```python
from build123d import *

# Parameters (mm, degrees)
SKETCH1_W                                         = 400
SKETCH1_H                                         = 560
BOSS_EXTRUDE1_DEPTH                               = 16
SKETCH2_W                                         = 30
SKETCH2_H                                         = 85
CUT_EXTRUDE1_DEPTH                                = 10
CHAMFER2_SIZE                                     = 10
F_8_36_TAPPED_HOLE1_AT_2_COUNT                    = 2
F_8_36_TAPPED_HOLE1_AT_2_PITCH                    = 31
F_8_36_TAPPED_HOLE1_AT_3_COUNT                    = 2
F_8_36_TAPPED_HOLE1_AT_3_PITCH                    = 62
LPATTERN1_COUNT                                   = 3
LPATTERN1_PITCH                                   = 160
CSK_FOR_8_FLAT_HEAD_MACHINE_SCREW_100_D           = 4.4958
CSK_FOR_8_FLAT_HEAD_MACHINE_SCREW_100_CSINK_D     = 8.4328
CSK_FOR_8_FLAT_HEAD_MACHINE_SCREW_100_CSINK_ANGLE = 100


with BuildPart() as part:
    # Sketch1 → Boss-Extrude1 (new body)
    with BuildSketch(Plane(origin=(0, 0, 0), x_dir=(1, 0, 0), z_dir=(0, 1, 0))):
        Rectangle(SKETCH1_W, SKETCH1_H)
    extrude(amount=BOSS_EXTRUDE1_DEPTH)

    # Sketch2 → Cut-Extrude1 (cut)
    with BuildSketch(Plane(origin=(0, 16, 0), x_dir=(1, 0, 0), z_dir=(0, 1, 0))):
        with Locations((-185, 160)):
            Rectangle(SKETCH2_W, SKETCH2_H)
        with Locations((-185, 0)):
            Rectangle(SKETCH2_W, SKETCH2_H)
        with Locations((-185, -160)):
            Rectangle(SKETCH2_W, SKETCH2_H)
    extrude(amount=-CUT_EXTRUDE1_DEPTH, mode=Mode.SUBTRACT)

    # Chamfer2
    chamfer2_edges = [part.edges().sort_by_distance(p)[0] for p in [
        (-200, 16, -241.25),
        (-200, 16, -80),
        (-200, 16, 80),
        (-200, 16, 241.25),
    ]]
    chamfer(chamfer2_edges, length=CHAMFER2_SIZE)

    # Sketch7 → #8-36 Tapped Hole1 (revolve, cut)
    with BuildSketch(Plane(origin=(-186, 6, 129), x_dir=(0, 0, 1), z_dir=(1, 0, 0))):
        Polygon((0, 0), (0, 26.037806461), (1.7272, 25), (1.7272, 0), align=None)
    f_8_36_tapped_hole1 = revolve(axis=Axis((-186, 12.35, 129), (0, -1, 0)), mode=Mode.SUBTRACT)

    # #8-36 Tapped Hole1 at 2: #8-36 Tapped Hole1 ×2
    with Locations(*[(0, 0, i * F_8_36_TAPPED_HOLE1_AT_2_PITCH) for i in range(1, F_8_36_TAPPED_HOLE1_AT_2_COUNT)]):
        add(f_8_36_tapped_hole1, mode=Mode.SUBTRACT)

    # #8-36 Tapped Hole1 at 3: #8-36 Tapped Hole1 ×2
    with Locations(*[(0, 0, i * F_8_36_TAPPED_HOLE1_AT_3_PITCH) for i in range(1, F_8_36_TAPPED_HOLE1_AT_3_COUNT)]):
        add(f_8_36_tapped_hole1, mode=Mode.SUBTRACT)

    # LPattern1: #8-36 Tapped Hole1 ×3
    with Locations(*[(0, 0, -i * LPATTERN1_PITCH) for i in range(1, LPATTERN1_COUNT)]):
        add(f_8_36_tapped_hole1, mode=Mode.SUBTRACT)

    # LPattern1 copy 1 sketch → LPattern1 copy 1 (revolve, cut)
    with BuildSketch(Plane(origin=(-186, 6, 0), x_dir=(0, 0, 1), z_dir=(1, 0, 0))):
        Polygon((0, 0), (0, 26.037806461), (1.7272, 25), (1.7272, 0), align=None)
    revolve(axis=Axis((-186, 12.35, 0), (0, -1, 0)), mode=Mode.SUBTRACT)

    # LPattern1 copy 2 sketch → LPattern1 copy 2 (revolve, cut)
    with BuildSketch(Plane(origin=(-186, 6, -160), x_dir=(0, 0, 1), z_dir=(1, 0, 0))):
        Polygon((0, 0), (0, 26.037806461), (1.7272, 25), (1.7272, 0), align=None)
    revolve(axis=Axis((-186, 12.35, -160), (0, -1, 0)), mode=Mode.SUBTRACT)

    # LPattern1 copy 3 sketch → LPattern1 copy 3 (revolve, cut)
    with BuildSketch(Plane(origin=(-186, 6, 31), x_dir=(0, 0, 1), z_dir=(1, 0, 0))):
        Polygon((0, 0), (0, 26.037806461), (1.7272, 25), (1.7272, 0), align=None)
    revolve(axis=Axis((-186, 12.35, 31), (0, -1, 0)), mode=Mode.SUBTRACT)

    # LPattern1 copy 4 sketch → LPattern1 copy 4 (revolve, cut)
    with BuildSketch(Plane(origin=(-186, 6, -129), x_dir=(0, 0, 1), z_dir=(1, 0, 0))):
        Polygon((0, 0), (0, 26.037806461), (1.7272, 25), (1.7272, 0), align=None)
    revolve(axis=Axis((-186, 12.35, -129), (0, -1, 0)), mode=Mode.SUBTRACT)

    # CSK for #8 Flat Head Machine Screw (100)1 (through all)
    with Locations(Plane(origin=(617.704940286, 16, 0), x_dir=(1, 0, 0), z_dir=(0, 1, 0))):
        with Locations((-447.704940286, -222), (-597.704940286, -222), (-747.704940286, -222)):
            csk_for_8_flat_head_machine_screw_100 = CounterSinkHole(CSK_FOR_8_FLAT_HEAD_MACHINE_SCREW_100_D / 2, CSK_FOR_8_FLAT_HEAD_MACHINE_SCREW_100_CSINK_D / 2, counter_sink_angle=CSK_FOR_8_FLAT_HEAD_MACHINE_SCREW_100_CSINK_ANGLE)

    # Mirror1: CSK for #8 Flat Head Machine Screw (100)1 across plane
    add(csk_for_8_flat_head_machine_screw_100.mirror(Plane.XY), mode=Mode.SUBTRACT)


solid = part.part
```
Could you check a few things on this model? Use its own coordinates, in mm. A direction names the side the tool comes from. Coordinates: 2 decimals unless noted, no trailing zeros. Write each loop counter-clockwise with the first axis right and the second up, starting at its lowest first coordinate (ties: lowest second). Pieces come first, ordered by that corner, then holes. Notation, with made-up numbers: (-21, 13.5) -> (-17, 13.5) arc R21 ccw to (-17, 44.5) -> close; hole circle Ø7 at (8, 24). An arc over 180 degrees is marked (long way). Return JSON: item names as keys, results as strings.
(1) We'd pull the mould along Z, two halves only. Please class faces 3 (the flat face through (2, 16, -4)), 4 (the flat face through (-3, 8, 280)), 5 (the flat face through (-182, 6, 159)): +Z half, -Z half, draft (parallel to the pull), parting line (faces both ways), or undercut.
Numbers:
{"face 3": "draft", "face 4": "+Z half", "face 5": "undercut"}
(2) I need wall thicknesses on L1, parallel to Z at x = -130, y = 10.5; L2, parallel to X at y = 11.25, z = -222; L3, parallel to X at y = 1.3, z = -160. Which ranges of each line are inside material? Lowest first, please.
Numbers:
{"L1": "z = -280 to -224.25, -219.75 to 219.75, 224.25 to 280", "L2": "x = -194.75 to -132.25, -127.75 to 17.75, 22.25 to 167.75, 172.25 to 200", "L3": "x = -200 to -187.73, -184.27 to 200"}
(3) Imagine slicing it at A-A, the plane y = 10. Please give me the cut outline in (x, z).
Numbers:
{"outline": "(-196, -280) -> (200, -280) -> (200, 280) -> (-196, 280) -> (-196, 202.5) -> (-170, 202.5) -> (-170, 117.5) -> (-196, 117.5) -> (-196, 42.5) -> (-170, 42.5) -> (-170, -42.5) -> (-196, -42.5) -> (-196, -117.5) -> (-170, -117.5) -> (-170, -202.5) -> (-196, -202.5) -> close; hole circle Ø4.5 at (-130, -222); hole circle Ø4.5 at (-130, 222); hole circle Ø4.5 at (20, -222); hole circle Ø4.5 at (20, 222); hole circle Ø4.5 at (170, -222); hole circle Ø4.5 at (170, 222)"}
(4) I'm going to push flat-ended pins straight in: pin 1 (3 mm diameter, centred on x = -186, z = 129, fed in from +Y); pin 2 (7 mm diameter, centred on x = 20, z = -222, fed in from +Y); pin 3 (6 mm diameter, centred on x = 170, z = 222, fed in from +Y); pin 4 (8 mm diameter, centred on y = 11.5, z = -173, fed in from -X). Where does each tip first touch, or does it pass through?
Numbers:
{"pin 1": "passes through", "pin 2": "stops at y = 15.4", "pin 3": "stops at y = 14.98", "pin 4": "stops at x = -170"}
(5) Which directions (+Z, -Z, +X, -X, +Y, -Y) give clear straight access to the entire face, cutting with the end or side of a thin tool? Please do faces 1 (the flat face through (-3, 0, -4)), 2 (the flat face through (-182, 6, -161)).
Numbers:
{"face 1": "+Z, -Z, +X, -X, -Y", "face 2": "-X, +Y"}
